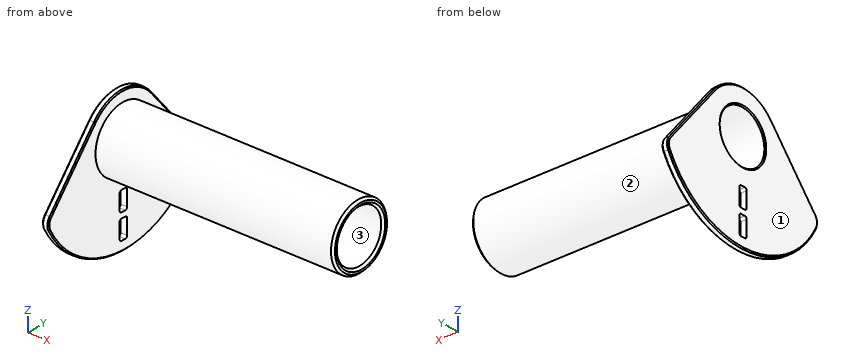
from build123d import *

# Parameters (mm, degrees)
SKETCH001_W     = 4
SKETCH001_H     = 9
POCKET_DEPTH    = 3
POCKET001_DEPTH = 5
FILLET_R        = 5
FILLET001_R     = 1
CHAMFER_SIZE    = 0.5
CHAMFER001_SIZE = 1


with BuildPart() as part:
    # Sketch → Revolution (revolve)
    with BuildSketch(Plane.XY):
        Polygon((0, 45), (3, 45), (3, 15), (115, 15), (115, 12.05), (0, 12.05), align=None)
    revolve(axis=Axis((0, 0, 0), (1, 0, 0)))

    # Sketch001 → Pocket (cut, symmetric)
    with BuildSketch(Plane.YZ.offset(2)):
        with Locations((0, -36)):
            Rectangle(SKETCH001_W, SKETCH001_H)
        with Locations((0, -24.5)):
            Rectangle(SKETCH001_W, SKETCH001_H)
    extrude(amount=POCKET_DEPTH, both=True, mode=Mode.SUBTRACT)

    # Sketch002 → Pocket001 (cut)
    with BuildSketch(Plane(origin=(0, 0, 0), x_dir=(0, -1, 0), z_dir=(-1, 0, 0))):
        with BuildLine():
            ThreePointArc((44.777118, -22.248814), (0, 50), (-44.777118, -22.248814))
            Line((-44.777118, -22.248814), (-15.320889, 12.855752))
            ThreePointArc((15.320889, 12.855752), (0, 20), (-15.320889, 12.855752))
            Line((15.320889, 12.855752), (44.777118, -22.248814))
        make_face()
    extrude(amount=-POCKET001_DEPTH, mode=Mode.SUBTRACT)

    # Fillet
    fillet_edges = [part.edges().sort_by_distance(p)[0] for p in [
        (1.5, 41.232486, -18.024487),
        (1.5, -41.232486, -18.024487),
    ]]
    fillet(fillet_edges, radius=FILLET_R)

    # Fillet001
    fillet001_edges = [part.edges().sort_by_distance(p)[0] for p in [
        (1.5, 2, -20),
        (1.5, -2, -20),
        (1.5, -2, -29),
        (1.5, 2, -29),
        (1.5, 2, -31.5),
        (1.5, -2, -31.5),
        (1.5, -2, -40.5),
        (1.5, 2, -40.5),
    ]]
    fillet(fillet001_edges, radius=FILLET001_R)

    # Chamfer
    chamfer_edges = [part.edges().sort_by_distance(p)[0] for p in [
        (0, 0, -45),
        (3, 0, -45),
        (0, -12.05, 0),
    ]]
    chamfer(chamfer_edges, length=CHAMFER_SIZE)

    # Chamfer001
    chamfer001_edges = [part.edges().sort_by_distance(p)[0] for p in [
        (115, -15, 0),
        (115, -12.05, 0),
    ]]
    chamfer(chamfer001_edges, length=CHAMFER001_SIZE)


solid = part.part
Can you work these out from the model? Positions are in its coordinate system, mm. Face numbers are marked on the shaded views. Give positions to 0.01 mm unless a question says otherwise; leave off trailing zeros. Write each loop counter-clockwise with the first axis right and the second up, starting at its lowest first coordinate (ties: lowest second). Pieces come first, ordered by that corner, then holes. Notation, with made-up numbers: (-36, 6) -> (-11, 6) arc R33 cw to (-11, 44) -> close; hole circle Ø11 at (-12, 17). An arc over 180 degrees is marked (long way). Answer as a JSON object with one key per item and string values. Group by question number.
Item 1: Suppose I cut it at B-B (x = 80). Please give me the cut outline in (y, z), plus the area to 3 significant figures.
Item 2: Suppose I cut it at A-A (z = 0). Please give me the cut outline in (x, y).
Item 3: I'm going to push flat-ended pins straight in: P1, Ø8, axis at y = -14.5, z = -20.5, coming from the +X side; P2, Ø0.6, axis at x = 1, y = 0, coming from the +Z side; P3, Ø2, axis at x = 1.5, y = 0, coming from the -Z side; P4, Ø8, axis at x = 44, y = 21, coming from the +Z side. Where does each tip first touch, or does it pass through?
Item 4: Please list where these lines run through material, in increasing order: line 1 (Z direction, x = 47, y = 0); line 2 (Y direction, x = 67.5, z = -0.5); line 3 (X direction, y = 4.5, z = -32). Write a range as [from, to].
Item 5: We'd pull the mould along Y, two halves only. Please class the marked faces 1, 2 and 3: +Y half, -Y half, draft (parallel to the pull), parting line (faces both ways), or undercut.
Findings:
{
 "1": {"outline": "circle Ø30 at (0, 0); hole circle Ø24.1 at (0, 0)", "area": "251 mm²"},
 "2": {"outline": "(0, -25.46) -> (0.5, -26.11) -> (2.5, -26.11) -> (3, -25.46) -> (3, -15) -> (114, -15) -> (115, -14) -> (115, -13.05) -> (114, -12.05) -> (0.5, -12.05) -> (0, -12.55) -> close; (0, 12.55) -> (0.5, 12.05) -> (114, 12.05) -> (115, 13.05) -> (115, 14) -> (114, 15) -> (3, 15) -> (3, 25.46) -> (2.5, 26.11) -> (0.5, 26.11) -> (0, 25.46) -> close"},
 "3": {"P1": "stops at x = 3", "P2": "stops at z = 20", "P3": "stops at z = -45", "P4": "passes through"},
 "4": {"line 1": "z = [-15, -12.05], [12.05, 15]", "line 2": "y = [-14.99, -12.04], [12.04, 14.99]", "line 3": "x = [0, 3]"},
 "5": {"face 1": "draft", "face 2": "parting line", "face 3": "undercut"}
}
